```python
from build123d import *

# Parameters (mm, degrees)
BOSS_EXTRU_1_DEPTH            = 20
ENL_V_MAT_EXTRU_2_DEPTH       = 324.482768921
ENL_V_MAT_EXTRU_2_DEPTH_BACK  = 249
ENL_V_MAT_EXTRU_3_DEPTH       = 324.482768921
ENL_V_MAT_EXTRU_3_DEPTH_BACK  = 249
ENL_V_MAT_EXTRU_4_DEPTH       = 316.090774845
ENL_V_MAT_EXTRU_4_DEPTH_BACK  = 219
ENL_V_MAT_EXTRU_5_DEPTH       = 316.090774845
ENL_V_MAT_EXTRU_5_DEPTH_BACK  = 219
ENL_V_MAT_EXTRU_7_DEPTH       = 316.090774845
ENL_V_MAT_EXTRU_7_DEPTH_BACK  = 219
ENL_V_MAT_EXTRU_8_DEPTH       = 316.090774845
ENL_V_MAT_EXTRU_8_DEPTH_BACK  = 219
ENL_V_MAT_EXTRU_9_DEPTH       = 324.482768921
ENL_V_MAT_EXTRU_9_DEPTH_BACK  = 249
ENL_V_MAT_EXTRU_10_DEPTH      = 324.482768921
ENL_V_MAT_EXTRU_10_DEPTH_BACK = 249


with BuildPart() as part:
    # Esquisse1 → Boss.-Extru.1 (new body)
    with BuildSketch(Plane.XY):
        Polygon((-33.910103697, 30.671339951), (215.089896303, 30.671339951), (215.089896303, 25.371339951), (220.389896303, 25.371339951), (220.389896303, -193.628660049), (215.089896303, -193.628660049), (215.089896303, -198.928660049), (-33.910103697, -198.928660049), (-33.910103697, -193.628660049), (-39.210103697, -193.628660049), (-39.210103697, 25.371339951), (-33.910103697, 25.371339951), align=None)
    extrude(amount=BOSS_EXTRU_1_DEPTH)

    # Esquisse2 → Enlèv. mat.-Extru.2 (cut, two sides: drawn at the far end of the back side and taken through both)
    with BuildSketch(Plane(origin=(215.089896303, 0, 0), x_dir=(0, 0, -1), z_dir=(1, 0, 0)).offset(-ENL_V_MAT_EXTRU_2_DEPTH_BACK)):
        Polygon((-489.896433994, 25.371339951), (-20, 25.371339951), (-12.45, 25.371339951), (-12.45, 26.921339951), (-16.15, 26.921339951), (-16.15, 27.921339951), (-12.65, 30.671339951), (356.838183396, 320.983484048), (47.072753092, 1208.257969711), (-799.661864298, 912.645825614), align=None)
    extrude(amount=ENL_V_MAT_EXTRU_2_DEPTH + ENL_V_MAT_EXTRU_2_DEPTH_BACK, mode=Mode.SUBTRACT)

    # Esquisse3 → Enlèv. mat.-Extru.3 (cut, two sides: drawn at the far end of the back side and taken through both)
    with BuildSketch(Plane(origin=(215.089896303, 0, 0), x_dir=(0, 0, -1), z_dir=(1, 0, 0)).offset(-ENL_V_MAT_EXTRU_3_DEPTH_BACK)):
        Polygon((469.896433994, 25.371339951), (0, 25.371339951), (-7.55, 25.371339951), (-7.55, 26.921339951), (-3.85, 26.921339951), (-3.85, 28.020478953), (-7.35, 30.671339951), (-381.934453377, 314.377430771), (-79.989898168, 1204.343789854), (771.840989202, 915.337699034), align=None)
    extrude(amount=ENL_V_MAT_EXTRU_3_DEPTH + ENL_V_MAT_EXTRU_3_DEPTH_BACK, mode=Mode.SUBTRACT)

    # Esquisse5 → Enlèv. mat.-Extru.4 (cut, two sides: drawn at the far end of the back side and taken through both)
    with BuildSketch(Plane(origin=(0, 25.371339951, 0), x_dir=(1, 0, 0), z_dir=(0, 1, 0)).offset(-ENL_V_MAT_EXTRU_4_DEPTH_BACK)):
        Polygon((215.089896303, 0), (215.089896303, -7.55), (216.639896303, -7.55), (216.639896303, -3.85), (217.639896303, -3.85), (220.389896303, -7.35), (220.389896303, 0), align=None)
    extrude(amount=ENL_V_MAT_EXTRU_4_DEPTH + ENL_V_MAT_EXTRU_4_DEPTH_BACK, mode=Mode.SUBTRACT)

    # Esquisse7 → Enlèv. mat.-Extru.5 (cut, two sides: drawn at the far end of the back side and taken through both)
    with BuildSketch(Plane(origin=(0, 25.371339951, 0), x_dir=(1, 0, 0), z_dir=(0, 1, 0)).offset(-ENL_V_MAT_EXTRU_5_DEPTH_BACK)):
        Polygon((547.721673026, 403.954079466), (220.389896303, -12.65), (217.639896303, -16.15), (216.639896303, -16.15), (216.639896303, -12.45), (215.089896303, -12.45), (215.089896303, -20), (215.089896303, -549.816054004), (1215.620408753, -898.755730707), (1548.252185476, 55.014402763), align=None)
    extrude(amount=ENL_V_MAT_EXTRU_5_DEPTH + ENL_V_MAT_EXTRU_5_DEPTH_BACK, mode=Mode.SUBTRACT)

    # Esquisse9 → Enlèv. mat.-Extru.7 (cut, two sides: drawn at the far end of the back side and taken through both)
    with BuildSketch(Plane(origin=(0, 25.371339951, 0), x_dir=(1, 0, 0), z_dir=(0, 1, 0)).offset(-ENL_V_MAT_EXTRU_7_DEPTH_BACK)):
        Polygon((-33.910103697, -20), (-33.910103697, -12.45), (-35.460103697, -12.45), (-35.460103697, -16.15), (-36.460103697, -16.15), (-39.210103697, -12.65), (-39.210103697, -20), align=None)
    extrude(amount=ENL_V_MAT_EXTRU_7_DEPTH + ENL_V_MAT_EXTRU_7_DEPTH_BACK, mode=Mode.SUBTRACT)

    # Esquisse10 → Enlèv. mat.-Extru.8 (cut, two sides: drawn at the far end of the back side and taken through both)
    with BuildSketch(Plane(origin=(0, 25.371339951, 0), x_dir=(1, 0, 0), z_dir=(0, 1, 0)).offset(-ENL_V_MAT_EXTRU_8_DEPTH_BACK)):
        Polygon((-366.54188042, -423.954079466), (-39.210103697, -7.35), (-36.460103697, -3.85), (-35.460103697, -3.85), (-35.460103697, -7.55), (-33.910103697, -7.55), (-33.910103697, 0), (-33.910103697, 529.816054004), (-1034.440616146, 878.755730707), (-1367.072392869, -75.014402763), align=None)
    extrude(amount=ENL_V_MAT_EXTRU_8_DEPTH + ENL_V_MAT_EXTRU_8_DEPTH_BACK, mode=Mode.SUBTRACT)

    # Esquisse12 → Enlèv. mat.-Extru.9 (cut, two sides: drawn at the far end of the back side and taken through both)
    with BuildSketch(Plane.ZY.offset(33.910103697).offset(-ENL_V_MAT_EXTRU_9_DEPTH_BACK)):
        Polygon((20, -193.628660049), (12.45, -193.628660049), (12.45, -195.178660049), (16.15, -195.178660049), (16.15, -196.178660049), (12.65, -198.928660049), (20, -198.928660049), align=None)
    extrude(amount=ENL_V_MAT_EXTRU_9_DEPTH + ENL_V_MAT_EXTRU_9_DEPTH_BACK, mode=Mode.SUBTRACT)

    # Esquisse13 → Enlèv. mat.-Extru.10 (cut, two sides: drawn at the far end of the back side and taken through both)
    with BuildSketch(Plane.ZY.offset(33.910103697).offset(-ENL_V_MAT_EXTRU_10_DEPTH_BACK)):
        Polygon((376.838183396, -489.240804146), (7.35, -198.928660049), (3.85, -196.178660049), (3.85, -195.178660049), (7.55, -195.178660049), (7.55, -193.628660049), (0, -193.628660049), (-469.896433994, -193.628660049), (-779.661864298, -1080.903145712), (67.072753092, -1376.515289809), align=None)
    extrude(amount=ENL_V_MAT_EXTRU_10_DEPTH + ENL_V_MAT_EXTRU_10_DEPTH_BACK, mode=Mode.SUBTRACT)


solid = part.part
```
Verification items for the finished model (mm, model axes). A direction names the side the tool comes from. Round coordinates to 2 decimals unless told otherwise and drop trailing zeros. Write each loop counter-clockwise with the first axis right and the second up, starting at its lowest first coordinate (ties: lowest second). Pieces come first, ordered by that corner, then holes.
1. Scan lines: L1, parallel to Y at x = 81, z = 15; L2, parallel to X at y = -132.5, z = 4; L3, parallel to X at y = -185.5, z = 4.25. Record each from-to range of solid material in increasing order.
2. Access from +Z, -Z, +X, -X, +Y, -Y to the whole of each face (thin tool, end or side, straight path). Record for faces 5 (the flat face through (-33.91, -86, 4)), 6 (the flat face through (-37, -193.629, 10)), 7 (the flat face through (218, 25.371, 10)), 8 (the flat face through (89, 25.371, 4)), 9 (the flat face through (-37, 25.371, 10)).
3. Section check B-B on x = 154. Enter the section's corners in (y, z), plus the area to 3 significant figures.
4. Section check A-A on y = -59.5. Enter the section's corners in (x, z).
5. Gauge pin test, flat ends, axial feed: P1, Ø3, axis at y = -53.5, z = 14.5, coming from the -X side; P2, Ø2.5, axis at y = -196, z = 9, coming from the +X side; P3, Ø1.1, axis at x = 80.5, z = 5.5, coming from the -Y side. Record the tip position at first contact, or that the pin passes through.
6. Draft check along X on faces 1 (the flat face through (92, -83, 20)), 2 (the flat face through (215.09, 28, 10)), 3 (the flat face through (215.09, -86, 16)), 4 (the flat face through (-33.91, -86, 16)). Enter one of: +X half, -X half, draft (parallel to the pull), parting line (faces both ways), or undercut.
Answer:
1. L1: y = -197.08 to -195.18, -193.63 to 25.37, 26.92 to 28.82
1. L2: x = -36.58 to -35.46, -33.91 to 215.09, 216.64 to 217.76
1. L3: x = -36.77 to -35.46, -33.91 to 215.09, 216.64 to 217.95
2. face 5: -Z, +Y, -Y
2. face 6: +Z, -Z, -X, -Y
2. face 7: +Z, -Z, +X, +Y
2. face 8: -Z, +X, -X
2. face 9: +Z, -Z, -X, +Y
3. outline: (-198.93, 7.35) - (-196.18, 3.85) - (-195.18, 3.85) - (-195.18, 7.55) - (-193.63, 7.55) - (-193.63, 0) - (25.37, 0) - (25.37, 7.55) - (26.92, 7.55) - (26.92, 3.85) - (28.02, 3.85) - (30.67, 7.35) - (30.67, 12.65) - (27.92, 16.15) - (26.92, 16.15) - (26.92, 12.45) - (25.37, 12.45) - (25.37, 20) - (-193.63, 20) - (-193.63, 12.45) - (-195.18, 12.45) - (-195.18, 16.15) - (-196.18, 16.15) - (-198.93, 12.65) - close
3. area: 4,470 mm2
4. outline: (-39.21, 7.35) - (-36.46, 3.85) - (-35.46, 3.85) - (-35.46, 7.55) - (-33.91, 7.55) - (-33.91, 0) - (215.09, 0) - (215.09, 7.55) - (216.64, 7.55) - (216.64, 3.85) - (217.64, 3.85) - (220.39, 7.35) - (220.39, 12.65) - (217.64, 16.15) - (216.64, 16.15) - (216.64, 12.45) - (215.09, 12.45) - (215.09, 20) - (-33.91, 20) - (-33.91, 12.45) - (-35.46, 12.45) - (-35.46, 16.15) - (-36.46, 16.15) - (-39.21, 12.65) - close
5. P1: stops at x = -38.94
5. P2: stops at x = 215.09
5. P3: stops at y = -197.91
6. face 1: draft
6. face 2: +X half
6. face 3: undercut
6. face 4: undercut
